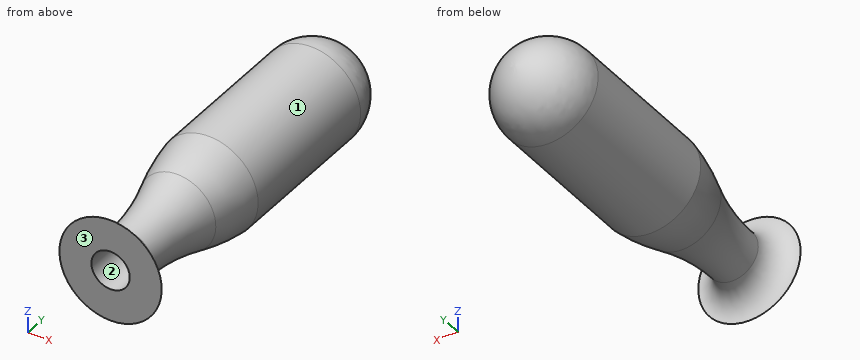
```python
from build123d import *

# Parameters (mm, degrees)
CROQUIS2_R            = 1.5
CORTAR_EXTRUIR1_DEPTH = 10


with BuildPart() as part:
    # Croquis1 → Revolución1 (revolve)
    with BuildSketch(Plane.XY, mode=Mode.PRIVATE) as revoluci_n1_sk:
        with BuildLine():
            Line((0, -5.810793785), (0, 22.186814978))
            ThreePointArc((0, 22.186814978), (2.738614464, 20.96831032), (3.861709813, 18.189206215))
            Line((3.861709813, 18.189206215), (3.861709813, 5.931416864))
            ThreePointArc((3.861709813, 5.931416864), (3.528216573, 4.037892304), (3, 2.189206215))
            ThreePointArc((3, 2.189206215), (2.251712409, -0.76941252), (2, -3.810793785))
            ThreePointArc((2, -3.810793785), (2.585786438, -5.225007347), (4, -5.810793785))
            Line((4, -5.810793785), (0, -5.810793785))
        make_face()
    revolve(revoluci_n1_sk.sketch.rotate(Axis((0, -5.810793785, 0), (0, 1, 0)), 90), axis=Axis((0, -5.810793785, 0), (0, 1, 0)))

    # Croquis2 → Cortar-Extruir1 (cut)
    with BuildSketch(Plane.XZ.offset(5.810793785)):
        with Locations(Location((0, 0, 0), (0, 0, 270))):
            Circle(CROQUIS2_R)
    extrude(amount=-CORTAR_EXTRUIR1_DEPTH, mode=Mode.SUBTRACT)


solid = part.part
```
Here's how the part is built. I have some questions about the finished solid (model axes, mm). Face numbers are marked on the shaded views. Round coordinates to 2 decimals unless told otherwise and drop trailing zeros. Order: outer loops, then holes, each group sorted by start corner. A loop starts at its lowest first (then second) coordinate and runs counter-clockwise, first axis right, second up. Notation, with made-up numbers: (46, 59) -> (84, 59) arc R17 cw to (84, 75) -> close; hole circle Ø6 at (6, 32.5). An arc over 180 degrees is marked (long way). Use a Markdown table: item, result. Add a question column.
(1) For pin 1 Ø4 at (y, z) = (18, 1.5) entering from +X; pin 2 Ø2.5 at (x, z) = (0.5, -0.5) entering from -Y; pin 3 Ø1.5 at (y, z) = (-3, 2.5) entering from +X, each with a flat end and sliding along its axis, tell me the tip position at first contact or that it passes through.
(2) I need wall thicknesses on line 1 along X through (y, z) = (0.25, 0); line 2 along Z through (x, y) = (-1, -0.5); line 3 along X through (y, z) = (2.25, 0). Which ranges of each line are inside material? Lowest first, please.
(3) Suppose I cut it at A-A, the plane y = 15.25. Please give me the cut outline in (x, z), and give its area (4 significant figures).
(4) Suppose I cut it at B-B, the plane y = -1.75. Please give me the cut outline in (x, z).
(5) If we mould it in two halves opening along Z, with no side actions, what happens to the marked faces 1, 2 and 3? For each: released by +Z, released by -Z, zero draft, split by the parting line, or undercut.
Verdict:
| question | item | result |
|---|---|---|
| 1 | pin 1 | x = 3.86 |
| 1 | pin 2 | y = -5.81 |
| 1 | pin 3 | x = 1.01 |
| 2 | line 1 | -2.45 to -1.5, 1.5 to 2.45 |
| 2 | line 2 | -2.07 to -1.12, 1.12 to 2.07 |
| 2 | line 3 | -3.02 to -1.5, 1.5 to 3.02 |
| 3 | outline | circle Ø7.72 at (0, 0) |
| 3 | area | 46.85 mm2 |
| 4 | outline | circle Ø4.23 at (0, 0); hole circle Ø3 at (0, 0) |
| 5 | face 1 | split by the parting line |
| 5 | face 2 | undercut |
| 5 | face 3 | zero draft |
